Geometry: final body of the model. Coordinates: model frame, mm. A direction names the side the tool comes from. Give positions to 0.01 mm unless a question says otherwise; leave off trailing zeros. Order: outer loops, then holes, each group sorted by start corner. A loop starts at its lowest first (then second) coordinate and runs counter-clockwise, first axis right, second up. Notation, with made-up numbers: (-34, 74.5) -> (-12, 74.5) arc R34 ccw to (-12, 107.5) -> close; hole circle Ø10 at (38, -27). An arc over 180 degrees is marked (long way). Answer in a Markdown table with one row per item. Add a question column.
Q1. Contact query for flat-ended pins moving along their axis: P1, Ø1.6, axis at x = 7.5, z = 5.5, coming from the +Y side; P2, Ø1.5, axis at x = 12.5, y = 2, coming from the +Z side. Output: stop coordinate, or through.
Q2. Cut plane C-C on y = 31. Return the cut outline in (x, z), and give its area (3 significant figures).
Q3. Cut plane B-B on x = 14.75. Return the cut outline in (y, z).
Q4. Line query: line 1 along Z through (x, y) = (6.5, 23.5); line 2 along Z through (x, y) = (6.25, 35); line 3 along Y through (x, z) = (11.25, 3). Output: solid intervals per line, ascending. Write a range as from..to.
Q5. Set-up query: faces 4 (the face through (10, 28, 2)), 5 (the face through (10, 3, 2)), 6 (the face through (10, 30, 6)). Return all of +Z, -Z, +X, -X, +Y, -Y with unobstructed straight access to the full face (end or side cutting, diameter ignored); none if empty.
Q6. Cut plane D-D on z = 3.25. Return the cut outline in (x, y), and give its area (3 significant figures).
Q7. Cut plane A-A on y = 11. Return the cut outline in (x, z).
Q8. Pull-direction query (Z, two-part tool) for faces 1 (the face through (10, 20, 5)), 2 (the face through (10, 0, 1)), 3 (the face through (9.86, 8.06, 5.75)); classes: +Z half, -Z half, draft (parallel to the pull), parting line (faces both ways), or undercut.
from build123d import *

# Parameters (mm, degrees)
F1_DEPTH = 20


with BuildPart() as f1:
    # F0 (on Right) → F1 (new body)
    with BuildSketch(Plane.YZ):
        with BuildLine():
            Line((0, 2), (0, 0))
            Line((0, 0), (45, 0))
            Line((45, 0), (45, 2))
            Line((45, 2), (10, 2))
            ThreePointArc((10, 2), (8.5, 3.5), (10, 5))
            Line((10, 5), (30, 5))
            Line((30, 5), (30, 6.5))
            Line((30, 6.5), (10, 6.5))
            ThreePointArc((10, 6.5), (8.041277, 5.73374), (7.122461, 3.841776))
            ThreePointArc((7.122461, 3.841776), (6.48585, 2.530911), (5.128729, 2))
            Line((5.128729, 2), (0, 2))
        make_face()
    extrude(amount=F1_DEPTH)


solid = f1.part
Completed:
| question | item | result |
|---|---|---|
| 1 | P1 | stops at y = 30 |
| 1 | P2 | stops at z = 2 |
| 2 | outline | (0, 0) -> (20, 0) -> (20, 2) -> (0, 2) -> close |
| 2 | area | 40.0 mm² |
| 3 | outline | (0, 0) -> (45, 0) -> (45, 2) -> (10, 2) arc R1.5 cw to (10, 5) -> (30, 5) -> (30, 6.5) -> (10, 6.5) arc R2.89 ccw to (7.12, 3.84) arc R2 cw to (5.13, 2) -> (0, 2) -> close |
| 4 | line 1 | z = 0..2, 5..6.5 |
| 4 | line 2 | z = 0..2 |
| 4 | line 3 | y = 6.86..8.59 |
| 5 | face 4 | +X, -X, +Y |
| 5 | face 5 | +Z, +X, -X, -Y |
| 5 | face 6 | +Z, +X, -X, +Y |
| 6 | outline | (0, 6.98) -> (20, 6.98) -> (20, 8.52) -> (0, 8.52) -> close |
| 6 | area | 30.8 mm² |
| 7 | outline | (0, 0) -> (20, 0) -> (20, 2) -> (0, 2) -> close; (0, 5) -> (20, 5) -> (20, 6.5) -> (0, 6.5) -> close |
| 8 | face 1 | undercut |
| 8 | face 2 | draft |
| 8 | face 3 | +Z half |
